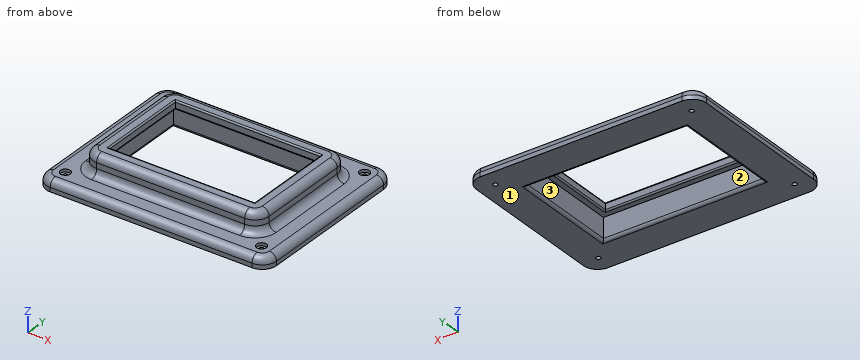
from build123d import *

# Parameters (mm, degrees)
SKETCH_1_W          = 162.6
SKETCH_1_H          = 124.2
SKETCH_1_R          = 1.6
SKETCH_1_W_2        = 102.6
SKETCH_1_H_2        = 64.2
EXTRUDE_1_DEPTH     = 22
SKETCH_2_R          = 3.5
CUT_EXTRUDE_1_DEPTH = 16
SKETCH_3_W          = 112.6
SKETCH_3_H          = 74.2
CUT_EXTRUDE_2_DEPTH = 16
SKETCH_4_W          = 162.6
SKETCH_4_H          = 124.2
SKETCH_4_W_2        = 124.6
SKETCH_4_H_2        = 86.2
CUT_EXTRUDE_3_DEPTH = 14
FILLET_1_R          = 10
FILLET_2_R          = 5
FILLET_3_R          = 1
FILLET_4_R          = 2
FILLET_5_R          = 1
FILLET_6_R          = 5


with BuildPart() as part:
    # 스케치1 → 보스-돌출1 (new body)
    with BuildSketch(Plane.XY):
        Rectangle(SKETCH_1_W, SKETCH_1_H)
        with Locations((-69.3, -50.1)):
            Circle(SKETCH_1_R, mode=Mode.SUBTRACT)
        with Locations((69.3, -50.1)):
            Circle(SKETCH_1_R, mode=Mode.SUBTRACT)
        with Locations((69.3, 50.1)):
            Circle(SKETCH_1_R, mode=Mode.SUBTRACT)
        with Locations((-69.3, 50.1)):
            Circle(SKETCH_1_R, mode=Mode.SUBTRACT)
        Rectangle(SKETCH_1_W_2, SKETCH_1_H_2, mode=Mode.SUBTRACT)
    extrude(amount=EXTRUDE_1_DEPTH)

    # 스케치2 → 컷-돌출1 (cut)
    with BuildSketch(Plane.XY.offset(22)):
        with Locations((-69.3, 50.1)):
            Circle(SKETCH_2_R)
        with Locations((69.3, 50.1)):
            Circle(SKETCH_2_R)
        with Locations((69.3, -50.1)):
            Circle(SKETCH_2_R)
        with Locations((-69.3, -50.1)):
            Circle(SKETCH_2_R)
    extrude(amount=-CUT_EXTRUDE_1_DEPTH, mode=Mode.SUBTRACT)

    # 스케치3 → 컷-돌출2 (cut)
    with BuildSketch(Plane(origin=(0, 0, 0), x_dir=(-1, 0, 0), z_dir=(0, 0, -1))):
        Rectangle(SKETCH_3_W, SKETCH_3_H)
    extrude(amount=-CUT_EXTRUDE_2_DEPTH, mode=Mode.SUBTRACT)

    # 스케치4 → 컷-돌출3 (cut)
    with BuildSketch(Plane.XY.offset(22)):
        Rectangle(SKETCH_4_W, SKETCH_4_H)
        Rectangle(SKETCH_4_W_2, SKETCH_4_H_2, mode=Mode.SUBTRACT)
    extrude(amount=-CUT_EXTRUDE_3_DEPTH, mode=Mode.SUBTRACT)

    # 필렛1
    fillet_1_edges = [part.edges().sort_by_distance(p)[0] for p in [
        (62.3, 43.1, 15),
        (-62.3, 43.1, 15),
        (-81.3, 62.1, 4),
        (81.3, 62.1, 4),
        (81.3, -62.1, 4),
        (-81.3, -62.1, 4),
        (-62.3, -43.1, 15),
        (62.3, -43.1, 15),
    ]]
    fillet(fillet_1_edges, radius=FILLET_1_R)

    # 필렛2
    fillet_2_edges = [part.edges().sort_by_distance(p)[0] for p in [
        (0, -43.1, 22),
        (-62.3, 0, 22),
        (62.3, 0, 22),
        (0, 43.1, 22),
        (-59.371067812, -40.171067812, 22),
        (-59.371067812, 40.171067812, 22),
        (59.371067812, 40.171067812, 22),
        (59.371067812, -40.171067812, 22),
        (0, 62.1, 8),
        (81.3, 0, 8),
        (-81.3, 0, 8),
        (0, -62.1, 8),
        (-78.371067812, 59.171067812, 8),
        (-78.371067812, -59.171067812, 8),
        (78.371067812, -59.171067812, 8),
        (78.371067812, 59.171067812, 8),
    ]]
    fillet(fillet_2_edges, radius=FILLET_2_R)

    # 필렛3
    fillet_3_edges = [part.edges().sort_by_distance(p)[0] for p in [
        (-51.3, 0, 22),
        (0, -32.1, 22),
        (51.3, 0, 22),
        (0, 32.1, 22),
    ]]
    fillet(fillet_3_edges, radius=FILLET_3_R)

    # 필렛4
    fillet_4_edges = [part.edges().sort_by_distance(p)[0] for p in [
        (-56.3, 0, 0),
        (0, 37.1, 0),
        (56.3, 0, 0),
        (0, -37.1, 0),
    ]]
    fillet(fillet_4_edges, radius=FILLET_4_R)

    # 필렛5
    fillet_5_edges = [part.edges().sort_by_distance(p)[0] for p in [
        (0, 32.1, 16),
        (-51.3, 0, 16),
        (0, -32.1, 16),
        (51.3, 0, 16),
    ]]
    fillet(fillet_5_edges, radius=FILLET_5_R)

    # 필렛6
    fillet_6_edges = [part.edges().sort_by_distance(p)[0] for p in [
        (0, -43.1, 8),
        (62.3, 0, 8),
        (0, 43.1, 8),
        (-62.3, 0, 8),
        (59.371067812, -40.171067812, 8),
        (59.371067812, 40.171067812, 8),
        (-59.371067812, 40.171067812, 8),
        (-59.371067812, -40.171067812, 8),
    ]]
    fillet(fillet_6_edges, radius=FILLET_6_R)


solid = part.part
Model file for the job. Use its own axes, mm. Face numbers are marked on the shaded views. Coordinates: 2 decimals unless noted, no trailing zeros. Write each loop counter-clockwise with the first axis right and the second up, starting at its lowest first coordinate (ties: lowest second). Pieces come first, ordered by that corner, then holes. Notation, with made-up numbers: (9.25, -23.5) -> (45.25, -23.5) arc R28 ccw to (45.25, 15.5) -> close; hole circle Ø6 at (-29, 44). An arc over 180 degrees is marked (long way). One line per item, written item: value. Start each with the question number.
1) Probe probe 1 along Y at (x, z) = (69.3, 7.05); probe 2 along X at (y, z) = (50.1, 1.45); probe 3 along Z at (x, y) = (-10, 35). List the from-to ranges inside material, lowest first.
2) Flat gauge pins, fed straight in: pin 1 Ø1.5 at (x, z) = (30.5, 18.5) entering from +Y; pin 2 Ø2 at (x, y) = (69, 48.5) entering from +Z; pin 3 Ø7 at (y, z) = (1, 9) entering from +X; pin 4 Ø22.5 at (x, y) = (4.5, -16) entering from -Z. Where does each tip first touch, or does it go through?
3) Slice it at A-A on x = 21. Write the cut outline in (y, z).
4) Pull direction X, two halves, no side cores. Call the marked faces 1, 2 and 3: +X half, -X half, draft (parallel to the pull), parting line (faces both ways), or undercut.
5) Slice it at B-B on y = 14.5. Write the cut outline in (x, z).
Answers follow:
1. probe 1: -60.03 to -53.6, -46.6 to 46.6, 53.6 to 60.03
1. probe 2: -81.3 to -70.9, -67.7 to 67.7, 70.9 to 81.3
1. probe 3: 16 to 22
2. pin 1: y = 43.04
2. pin 2: z = 6
2. pin 3: x = 80.63
2. pin 4: through
3. outline: (-62.1, 0) -> (-39.1, 0) arc R2 ccw to (-37.1, 2) -> (-37.1, 16) -> (-33.1, 16) arc R1 ccw to (-32.1, 17) -> (-32.1, 21) arc R1 ccw to (-33.1, 22) -> (-38.1, 22) arc R5 ccw to (-43.1, 17) -> (-43.1, 13) arc R5 cw to (-48.1, 8) -> (-57.1, 8) arc R5 ccw to (-62.1, 3) -> close; (32.1, 17) arc R1 ccw to (33.1, 16) -> (37.1, 16) -> (37.1, 2) arc R2 ccw to (39.1, 0) -> (62.1, 0) -> (62.1, 3) arc R5 ccw to (57.1, 8) -> (48.1, 8) arc R5 cw to (43.1, 13) -> (43.1, 17) arc R5 ccw to (38.1, 22) -> (33.1, 22) arc R1 ccw to (32.1, 21) -> close
4. face 1: draft
4. face 2: undercut
4. face 3: undercut
5. outline: (-81.3, 0) -> (-58.3, 0) arc R2 ccw to (-56.3, 2) -> (-56.3, 16) -> (-52.3, 16) arc R1 ccw to (-51.3, 17) -> (-51.3, 21) arc R1 ccw to (-52.3, 22) -> (-57.3, 22) arc R5 ccw to (-62.3, 17) -> (-62.3, 13) arc R5 cw to (-67.3, 8) -> (-76.3, 8) arc R5 ccw to (-81.3, 3) -> close; (51.3, 17) arc R1 ccw to (52.3, 16) -> (56.3, 16) -> (56.3, 2) arc R2 ccw to (58.3, 0) -> (81.3, 0) -> (81.3, 3) arc R5 ccw to (76.3, 8) -> (67.3, 8) arc R5 cw to (62.3, 13) -> (62.3, 17) arc R5 ccw to (57.3, 22) -> (52.3, 22) arc R1 ccw to (51.3, 21) -> close
